Could you check a few things on this model? Use its own coordinates, in mm. A direction names the side the tool comes from. Give positions to 0.01 mm unless a question says otherwise; leave off trailing zeros. Loops run counter-clockwise (first coordinate to the right, second up) from the corner with the lowest first, then second, coordinate; pieces in that order, holes last. Notation, with made-up numbers: (-10.5, -9) - (2.5, -9) arc R37 cw to (2.5, 27) - close; hole circle Ø2 at (53, 70). An arc over 180 degrees is marked (long way). One line per item, written item: value. Start each with the question number.
Q1. I'm going to push flat-ended pins straight in: P1, Ø0.6, axis at y = 49.5, z = -16, coming from the -X side; P2, Ø7, axis at x = 0, z = -4.5, coming from the +Y side; P3, Ø1.9, axis at x = 0, z = -4, coming from the -Y side; P4, Ø1.5, axis at x = 0.5, y = 49, coming from the +Z side. Where does each tip first touch, or does it pass through?
Q2. I want a section at D-D (z = -12). Please give me the cut outline in (x, y), then the cut area to 3 significant figures.
Q3. I want a section at A-A (z = 0). Please give me the cut outline in (x, y), then the cut area to 3 significant figures.
Q4. I want a section at B-B (x = 3). Please give me the cut outline in (y, z).
Q5. If we mould it in two halves opening along Z, with no side actions, what happens to faces 5 (the face through (-1.25, 0.75, 4.51)), 6 (the face through (1, 50.5, -16)), 7 (the face through (1, 50, -17.78))? For each: released by +Z, released by -Z, zero draft, split by the parting line, or undercut.
Q6. If I drill on line 1 (Z direction, x = 5.5, y = 0); line 2 (X direction, y = 15.5, z = -9.5); line 3 (Z direction, x = 16, y = 4), over which ranges is the centre line in solid material (lowest first)? Write a range as from..to.
Q7. For faces 1 (the face through (1, 50, 17.78)), 2 (the face through (9.767, -0.991, 4.463)), 3 (the face through (-1, -1.454, 0)), 4 (the face through (1, 50, -14.859)), which set-ups out of +Z, -Z, +X, -X, +Y, -Y let a thin tool reach every point of the face, with its end or its side?
Q8. I want a section at C-C (y = 38.5). Please give me the cut outline in (x, z), then the cut area to 3 significant figures.
Autodesk Inventor part; units mm, degrees
ref_plane "YZ Plane" through (0, 0, 0) normal (1, 0, 0) x (0, 1, 0)
ref_plane "XZ Plane" through (0, 0, 0) normal (0, 1, 0) x (-1, 0, 0)
ref_plane "XY Plane" through (0, 0, 0) normal (0, 0, 1) x (1, 0, 0)
sketch "Sketch1" plane through (0, 0, 0) normal (1, 0, 0) x (0, 1, 0)
  circle A0 centre (0, 0) radius 4.572
  circle A1 centre (0, 0) radius 8.382
  dimension "d0" = 9.144
  dimension "d1" = 3.81
extrude "Extrusion1" add sketch "Sketch1" along normal blind 19.812
sketch "Sketch2" plane through (0, 0, 0) normal (-1, 0, 0) x (0, 0, 1)
  circle A0 centre (0, 0) radius 8.382
  circle A1 centre (0, 0) radius 7.747
  circle A2 centre (0, 0) radius 8.382
  dimension "d42" = 0
extrude "Extrusion2" add sketch "Sketch2" along normal blind 2.54 contours A0 | A1
sketch "Sketch3" plane through (-2.54, 0, 0) normal (-1, 0, 0) x (0, 0, 1)
  line L0 (19.05, 48.5955) -> (-19.05, 48.5955)
  circle A0 centre (0, 0) radius 8.382
  line L1 (8.382, 0) -> (19.05, 48.5955)
  line L2 (-8.382, 0) -> (-19.05, 48.5955)
  arc A1 (8.382, 0) -> (-8.382, 0) centre (0, 0) ccw
  line L3 (-14.3129, 44.7855) -> (14.3129, 44.7855)
  line L4 (14.3129, 44.7855) -> (6.7152, 10.176)
  arc A2 (6.7152, 10.176) -> (-6.7152, 10.176) centre (0, 0) ccw
  line L5 (-6.7152, 10.176) -> (-14.3129, 44.7855)
  dimension "d6" = 38.1
  dimension "d7" = 19.05
  dimension "d8" = 3.81
extrude "Extrusion3" add sketch "Sketch3" against normal blind 6.35 contours L1 A0 L2 L0
sketch "Sketch6" plane through (-2.54, 44.7855, -14.3129) normal (0, -1, 0) x (1, 0, 0)
  line L0 (6.35, 32.4159) -> (26.9875, 32.4159)
  line L1 (13.4874, 32.4159) -> (13.4874, 26.0989)
  line L2 (26.9875, 32.4159) -> (26.9875, -3.9117)
  point P0 (2.54, 14.3129)
  dimension "d20" = 13.5001
sketch "Sketch10" plane through (0, 0, 0) normal (1, 0, 0) x (0, 0, -1)
  circle A0 centre (0, 0) radius 1.4542
  line L0 (-4.572, 1.4542) -> (4.572, 1.4542)
  line L1 (4.572, 1.4542) -> (4.572, -1.4542)
  line L2 (4.572, -1.4542) -> (-4.572, -1.4542)
  line L3 (-4.572, -1.4542) -> (-4.572, 1.4542)
  circle A1 centre (0, 0) radius 4.572
  dimension "d43" = 0
  dimension "d44" = 0
extrude "Extrusion7" cut sketch "Sketch10" against normal blind 22.225 contours A0 | A0 L0 A1 L2 | A0 L2 A1 L0 | A1 L3 L0 | L0 L1 A1 | A1 L1 L2 | L2 L3 A1
sketch "Sketch13" plane through (-2.54, 48.5955, 19.05) normal (0, 1, 0) x (1, 0, 0)
  line L0 (4.6355, 36.83) -> (1.7145, 36.83)
  line L1 (1.7145, 36.83) -> (1.7145, 33.909)
  line L2 (1.7145, 33.909) -> (4.6355, 33.909)
  line L3 (4.6355, 33.909) -> (4.6355, 36.83)
  line L4 (6.35, 38.1) -> (6.35, 0)
  line L5 (0, 38.1) -> (6.35, 38.1)
  line L6 (4.6228, 4.191) -> (1.7018, 4.191)
  line L7 (1.7018, 4.191) -> (1.7018, 1.27)
  line L8 (1.7018, 1.27) -> (4.6228, 1.27)
  line L9 (4.6228, 1.27) -> (4.6228, 4.191)
  line L10 (0, 0) -> (6.35, 0)
  point P0 (2.54, 19.05)
  dimension "d32" = 2.921
  dimension "d33" = 2.921
  dimension "d34" = 1.7145
  dimension "d35" = 1.27
  dimension "d36" = 2.921
  dimension "d37" = 2.921
  dimension "d38" = 1.7272
  dimension "d39" = 1.27
extrude "Extrusion9" add sketch "Sketch13" along normal blind 1.905
sketch "Sketch14" plane through (0, 0, 0) normal (-1, 0, 0) x (0, 0, 1)
  arc A0 (4.3346, -1.4542) -> (4.572, 0) centre (0, 0) ccw
  line L0 (4.3346, -1.4542) -> (4.572, -1.4542)
  line L1 (4.572, -1.4542) -> (4.572, 0)
  arc A1 (4.572, 0) -> (4.3346, 1.4542) centre (0, 0) ccw
  line L2 (4.572, 0) -> (4.572, 1.4542)
  line L3 (4.572, 1.4542) -> (4.3346, 1.4542)
  arc A2 (-4.572, 0) -> (-4.3346, -1.4542) centre (0, 0) ccw
  line L4 (-4.572, 0) -> (-4.572, -1.4542)
  line L5 (-4.572, -1.4542) -> (-4.3346, -1.4542)
  arc A3 (-4.3346, 1.4542) -> (-4.572, 0) centre (0, 0) ccw
  line L6 (-4.3346, 1.4542) -> (-4.572, 1.4542)
  line L7 (-4.572, 1.4542) -> (-4.572, 0)
extrude "Extrusion10" add sketch "Sketch14" along normal blind 2.54
properties part number "BasicThrustMotorHousingJustMotor"
Worked answers:
1. P1: stops at x = -0.83
1. P2: stops at y = 48.6
1. P3: stops at y = -7.81
1. P4: stops at z = 19.05
2. outline: (-2.54, 16.48) - (3.81, 16.48) - (3.81, 34.25) - (-2.54, 34.25) - close; (-2.54, 44.79) - (3.81, 44.79) - (3.81, 48.6) - (-2.54, 48.6) - close
2. area: 137 mm²
3. outline: (-2.54, -8.38) - (19.81, -8.38) - (19.81, -4.57) - (0, -4.57) - (0, -1.45) - (-2.54, -1.45) - close; (-2.54, 1.45) - (0, 1.45) - (0, 4.57) - (19.81, 4.57) - (19.81, 8.38) - (3.81, 8.38) - (3.81, 12.19) - (-2.54, 12.19) - close; (-2.54, 44.79) - (3.81, 44.79) - (3.81, 48.6) - (-2.54, 48.6) - close
3. area: 235 mm²
4. outline: (0, -8.38) - (48.6, -19.05) - (48.6, 19.05) - (0, 8.38) arc R8.38 ccw to start; hole circle Ø9.14 at (0, 0); hole (10.18, -6.72) - (44.79, -14.31) - (44.79, 14.31) - (10.18, 6.72) arc R12.19 cw to start
5. face 5: undercut
5. face 6: zero draft
5. face 7: released by -Z
6. line 1: z = -8.38..-4.57, 4.57..8.38
6. line 2: x = -2.54..3.81
6. line 3: z = -7.37..-2.21, 2.21..7.37
7. face 1: +Z, +X, -X, +Y
7. face 2: +X
7. face 3: +X, -X
7. face 4: +X, -X, +Y
8. outline: (-2.54, -16.83) - (3.81, -16.83) - (3.81, -12.93) - (-2.54, -12.93) - close; (-2.54, 12.93) - (3.81, 12.93) - (3.81, 16.83) - (-2.54, 16.83) - close
8. area: 49.5 mm²
